Verification items for the finished model (mm, model axes). Face numbers are marked on the shaded views. A direction names the side the tool comes from. Round coordinates to 2 decimals unless told otherwise and drop trailing zeros. Write each loop counter-clockwise with the first axis right and the second up, starting at its lowest first coordinate (ties: lowest second). Pieces come first, ordered by that corner, then holes. Notation, with made-up numbers: (57.5, 85) - (92.5, 85) arc R33 ccw to (92.5, 116) - close; hole circle Ø6 at (7.25, 69.25). An arc over 180 degrees is marked (long way). Answer as a JSON object with one key per item and string values.
```python
from build123d import *

# Parameters (mm, degrees)
F0_R     = 17
F1_DEPTH = 25
F3_D     = 9
F3_DEPTH = 17
F3_TIP   = 2.7038727856
F4_R     = 12.05
F5_DEPTH = 5
F6_SIZE  = 0.2


with BuildPart() as f1:
    # F0 (on Top) → F1 (new body)
    with BuildSketch(Plane.XY):
        Circle(F0_R)
    extrude(amount=F1_DEPTH)

    # F3
    with Locations(Plane(origin=(0, 0, 0), x_dir=(1, 0, 0), z_dir=(0, 0, -1))):
        with Locations((0, 0)):
            Hole(F3_D / 2, depth=F3_DEPTH)
            with Locations((0, 0, -(F3_DEPTH + F3_TIP / 2))):  # 118° drill point
                Cone(0, F3_D / 2, F3_TIP, mode=Mode.SUBTRACT)

    # F4 (on face) → F5 (cut)
    with BuildSketch(Plane.XY.offset(25)):
        Circle(F4_R)
    extrude(amount=-F5_DEPTH, mode=Mode.SUBTRACT)

    # F6
    f6_edges = [f1.edges().sort_by_distance(p)[0] for p in [
        (-17, 0, 25),
        (-12.05, 0, 25),
        (-17, 0, 0),
        (-4.5, 0, 0),
    ]]
    chamfer(f6_edges, length=F6_SIZE)


solid = f1.part
```
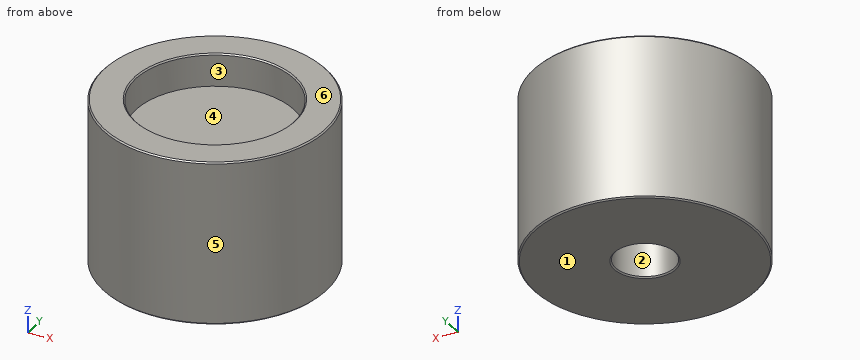
1. Material ranges on probe 1 along Y at (x, z) = (0, 21.75); probe 2 along Y at (x, z) = (0, 5); probe 3 along Z at (x, y) = (7, -9.5), recorded low to high. Write a range as from..to.
Completed:
{"probe 1": "y = -17..-12.05, 12.05..17", "probe 2": "y = -17..-4.5, 4.5..17", "probe 3": "z = 0..20"}
2. Mould release check, pull along Y, two halves, no side actions. Record for the marked faces 4, 5 and 6: released by +Y, released by -Y, zero draft, split by the parting line, or undercut.
Completed:
{"face 4": "undercut", "face 5": "split by the parting line", "face 6": "zero draft"}
3. Cross-section at A-A (z = 11.75). Record the boundary of the cut face in (x, y).
Completed:
{"outline": "circle Ø34 at (0, 0); hole circle Ø9 at (0, 0)"}
4. Access from +Z, -Z, +X, -X, +Y, -Y to the whole of each face (thin tool, end or side, straight path). Record for the marked faces 1, 2 and 3.
Completed:
{"face 1": "-Z, +X, -X, +Y, -Y", "face 2": "-Z", "face 3": "+Z"}
5. Go/stop test with flat-tipped pins: pin 1 (5 mm diameter, centred on y = 0.5, z = 16.5, fed in from +X); pin 2 (10 mm diameter, centred on y = -11.5, z = 18.5, fed in from -X); pin 3 (5.5 mm diameter, centred on x = 0, y = 0, fed in from +Z); pin 4 (8 mm diameter, centred on y = 5, z = 14.5, fed in from -X). Record where each tip stops, or that it passes through.
Completed:
{"pin 1": "stops at x = 17", "pin 2": "stops at x = -15.71", "pin 3": "stops at z = 20", "pin 4": "stops at x = -16.97"}
